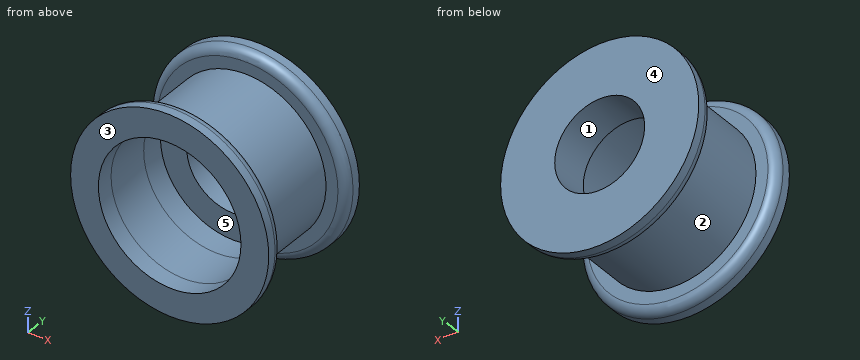
Autodesk Inventor part; units mm, degrees
ref_plane "YZ Plane" through (0, 0, 0) normal (1, 0, 0) x (0, 1, 0)
ref_plane "XZ Plane" through (0, 0, 0) normal (0, 1, 0) x (-1, 0, 0)
ref_plane "XY Plane" through (0, 0, 0) normal (0, 0, 1) x (1, 0, 0)
sketch "Boceto1" plane through (0, 0, 0) normal (0, 1, 0) x (-1, 0, 0)
  circle A0 centre (0, 0) radius 8.125
  circle A1 centre (0, 0) radius 8.925
  dimension "d0" = 16.25
  dimension "d1" = 0.8
extrude "Extrusión1" add sketch "Boceto1" along normal mid plane 10.3
sketch "Boceto2" plane through (0, 5.15, 0) normal (0, 1, 0) x (1, 0, 0)
  circle A0 centre (0, 0) radius 11.2887
  circle A1 centre (0, 0) radius 8.925
  circle A2 centre (0, 0) radius 8.125
extrude "Extrusión2" add sketch "Boceto2" along normal blind 2 contours A0 | A1
fillet "Empalme1" radius 1 1 edges at (-11.2887, 5.15, 0)
mirror "Simetría1" about plane through (0, 0, 0) normal (0, 1, 0) of "Extrusión2", "Empalme1"
sketch "Boceto3" plane through (0, 7.15, 0) normal (0, 1, 0) x (1, 0, 0)
  circle A0 centre (0, 0) radius 8.125
  circle A1 centre (0, 0) radius 5.125
  dimension "d7" = 10.25
extrude "Extrusión3" add sketch "Boceto3" against normal blind 4.515
properties part number "Roller"
Work out the finished part from the listing and answer in its coordinate system (mm). Face numbers are marked on the shaded views. A direction names the side the tool comes from. Round coordinates to 2 decimals unless told otherwise and drop trailing zeros. Write each loop counter-clockwise with the first axis right and the second up, starting at its lowest first coordinate (ties: lowest second). Pieces come first, ordered by that corner, then holes.
1) A cutting plane is placed at A-A on x = 0. Determine the outline of the cut face in (y, z) (3 decimals).
2) A cutting plane is placed at D-D on y = 6.75. Determine the outline of the cut face in (x, z) (3 decimals).
3) A cutting plane is placed at B-B on z = 0. Determine the outline of the cut face in (x, y) (3 decimals), and give its area (3 significant figures).
4) Determine the mould class of the marked faces 1, 2 and 3 for opening direction Z: pulls with the +Z half, pulls with the -Z half, needs draft (parallel to the pull), parting line crosses it, or undercut.
5) Which of the six approach directions +Z, -Z, +X, -X, +Y, -Y give full straight-line access (tool end or side, diameter ignored) to the marked faces 4 and 5?
6) Consider probe 1 along Y at (x, z) = (-8.25, -5.25); probe 2 along Z at (x, y) = (0, 1.35) (3 decimals); probe 3 along Z at (x, y) = (0, 3.9) (3 decimals). Determine where each line is inside the solid, lowest interval first.
7) A cutting plane is placed at C-C on y = 4.75. Determine the outline of the cut face in (x, z) (3 decimals), and give its area (3 significant figures).
8) Flat-ended cylindrical pins translate along their axes: P1, Ø13, axis at x = 0, z = 0, coming from the +Y side; P2, Ø6, axis at x = 2, z = -2.5, coming from the -Y side (3 decimals); P3, Ø2, axis at x = 7.5, y = -3, coming from the -Z side; P4, Ø1.5, axis at x = 0, y = 1, coming from the +Z side (3 decimals). Find the tip coordinate at first contact, or state that the pin passes through.
Entries:
1. outline: (-7.15, -11.289) - (-6.15, -11.289) arc R1 ccw to (-5.15, -10.289) - (-5.15, -8.925) - (5.15, -8.925) - (5.15, -10.289) arc R1 ccw to (6.15, -11.289) - (7.15, -11.289) - (7.15, -5.125) - (2.635, -5.125) - (2.635, -8.125) - (-7.15, -8.125) - close; (-7.15, 8.125) - (2.635, 8.125) - (2.635, 5.125) - (7.15, 5.125) - (7.15, 11.289) - (6.15, 11.289) arc R1 ccw to (5.15, 10.289) - (5.15, 8.925) - (-5.15, 8.925) - (-5.15, 10.289) arc R1 ccw to (-6.15, 11.289) - (-7.15, 11.289) - close
2. outline: circle Ø22.577 at (0, 0); hole circle Ø10.25 at (0, 0)
3. outline: (-11.289, -7.15) - (-8.125, -7.15) - (-8.125, 2.635) - (-5.125, 2.635) - (-5.125, 7.15) - (-11.289, 7.15) - (-11.289, 6.15) arc R1 ccw to (-10.289, 5.15) - (-8.925, 5.15) - (-8.925, -5.15) - (-10.289, -5.15) arc R1 ccw to (-11.289, -6.15) - close; (5.125, 2.635) - (8.125, 2.635) - (8.125, -7.15) - (11.289, -7.15) - (11.289, -6.15) arc R1 ccw to (10.289, -5.15) - (8.925, -5.15) - (8.925, 5.15) - (10.289, 5.15) arc R1 ccw to (11.289, 6.15) - (11.289, 7.15) - (5.125, 7.15) - close
3. area: 68.0 mm2
4. face 1: undercut
4. face 2: parting line crosses it
4. face 3: needs draft
5. face 4: +Z, -Z, +X, -X, +Y
5. face 5: -Y
6. probe 1: y = -7.15 to -5.15, 5.15 to 7.15
6. probe 2: z = -8.925 to -8.125, 8.125 to 8.925
6. probe 3: z = -8.925 to -5.125, 5.125 to 8.925
7. outline: circle Ø17.85 at (0, 0); hole circle Ø10.25 at (0, 0)
7. area: 168 mm2
8. P1: stops at y = 7.15
8. P2: stops at y = 2.635
8. P3: stops at z = -6.12
8. P4: stops at z = 8.925
